```python
from build123d import *

# Parameters (mm, degrees)
SKETCH_1_R          = 1.75
EXTRUDE_1_DEPTH     = 5
CUT_EXTRUDE_1_REACH = 7
SKETCH_2_W          = 35
SKETCH_2_H          = 3
SKETCH_3_W          = 8
SKETCH_3_H          = 8
CUT_EXTRUDE_3_DEPTH = 6


with BuildPart() as part:
    # 草圖1 → 填料-伸長1 (new body)
    with BuildSketch(Plane.XY):
        Polygon((-30, 16.5), (-30, 8.5), (-22, 8.5), (-22, -8.5), (-30, -8.5), (-30, -16.5), (30, -16.5), (30, -8.5), (22, -8.5), (22, 8.5), (30, 8.5), (30, 16.5), align=None)
        with Locations((-26, 12.5)):
            Circle(SKETCH_1_R, mode=Mode.SUBTRACT)
        with Locations((26, 12.5)):
            Circle(SKETCH_1_R, mode=Mode.SUBTRACT)
        with Locations((-26, -12.5)):
            Circle(SKETCH_1_R, mode=Mode.SUBTRACT)
        with Locations((26, -12.5)):
            Circle(SKETCH_1_R, mode=Mode.SUBTRACT)
    extrude(amount=EXTRUDE_1_DEPTH)

    # 草圖2 → 除料-伸長1 (cut, up to next)
    with BuildSketch(Plane.XY.offset(5), mode=Mode.PRIVATE) as cut_extrude_1_sk1:
        with Locations((0, -7)):
            Rectangle(SKETCH_2_W, SKETCH_2_H)
    cut_extrude_1_tool1 = extrude(cut_extrude_1_sk1.sketch, amount=-CUT_EXTRUDE_1_REACH, mode=Mode.PRIVATE) & part.part
    add(cut_extrude_1_tool1.solids().sort_by_distance((0, -7, 5))[0], mode=Mode.SUBTRACT)

    # 草圖3 → 除料-伸長3 (cut, through all)
    with BuildSketch(Plane.XY):
        with Locations((26, -12.5)):
            Rectangle(SKETCH_3_W, SKETCH_3_H)
    extrude(amount=CUT_EXTRUDE_3_DEPTH, mode=Mode.SUBTRACT)


solid = part.part
```
Design review of the part built by this model. Coordinates are the model's own, in mm. A direction names the side the tool comes from. Give positions to 0.01 mm unless a question says otherwise; leave off trailing zeros. Write each loop counter-clockwise with the first axis right and the second up, starting at its lowest first coordinate (ties: lowest second). Pieces come first, ordered by that corner, then holes.
(1) Add section D-D (x = 11). Give the boundary of the cut face in (y, z), and give its area (3 significant figures).
Checked values:
outline: (-16.5, 0) - (-8.5, 0) - (-8.5, 5) - (-16.5, 5) - close; (-5.5, 0) - (16.5, 0) - (16.5, 5) - (-5.5, 5) - close
area: 150 mm2
(2) Add section C-C (z = 0.55). Give the boundary of the cut face in (x, y).
Checked values:
outline: (-30, -16.5) - (22, -16.5) - (22, 8.5) - (30, 8.5) - (30, 16.5) - (-30, 16.5) - (-30, 8.5) - (-22, 8.5) - (-22, -8.5) - (-30, -8.5) - close; hole circle Ø3.5 at (-26, -12.5); hole circle Ø3.5 at (-26, 12.5); hole (-17.5, -8.5) - (17.5, -8.5) - (17.5, -5.5) - (-17.5, -5.5) - close; hole circle Ø3.5 at (26, 12.5)
(3) Add section B-B (x = -26). Give the boundary of the cut face in (y, z).
Checked values:
outline: (-16.5, 0) - (-14.25, 0) - (-14.25, 5) - (-16.5, 5) - close; (-10.75, 0) - (-8.5, 0) - (-8.5, 5) - (-10.75, 5) - close; (8.5, 0) - (10.75, 0) - (10.75, 5) - (8.5, 5) - close; (14.25, 0) - (16.5, 0) - (16.5, 5) - (14.25, 5) - close
(4) Tool access review of faces 5 (the face through (-30, 13, 2)), 6 (the face through (0, 0, 0)), 7 (the face through (-22, 0, 2)), 8 (the face through (-17.5, -7, 3)), 9 (the face through (22, -4, 2)): name each direction out of +Z, -Z, +X, -X, +Y, -Y from which nothing blocks a thin tool from reaching the whole face with its end or side.
Checked values:
face 5: +Z, -Z, -X, +Y, -Y
face 6: -Z, +X, -X, +Y, -Y
face 7: +Z, -Z, -X
face 8: +Z, -Z
face 9: +Z, -Z, +X, -Y
(5) Wall thickness on line 1 along Y through (x, z) = (-26, 1.7); line 2 along Y through (x, z) = (-23.5, 3.55); line 3 along Y through (x, z) = (2, 1.75): over which ranges is each line inside the solid? List them lowest first.
Checked values:
line 1: y = -16.5 to -14.25, -10.75 to -8.5, 8.5 to 10.75, 14.25 to 16.5
line 2: y = -16.5 to -8.5, 8.5 to 16.5
line 3: y = -16.5 to -8.5, -5.5 to 16.5
(6) Add section A-A (y = -12.5). Give the boundary of the cut face in (x, z), and give its area (4 significant figures).
Checked values:
outline: (-30, 0) - (-27.75, 0) - (-27.75, 5) - (-30, 5) - close; (-24.25, 0) - (22, 0) - (22, 5) - (-24.25, 5) - close
area: 242.5 mm2
(7) Mouldability with a two-part tool opening along Y and no side actions: class faces 1 (the face through (0, 16.5, 2)), 2 (the face through (0, 0, 5)), 3 (the face through (0, -5.5, 3)), 4 (the face through (-4, -16.5, 2)) as +Y half, -Y half, draft (parallel to the pull), parting line (faces both ways), or undercut.
Checked values:
face 1: +Y half
face 2: draft
face 3: undercut
face 4: -Y half
(8) Clearance check with flat-ended pins moving along their axes: pin 1 Ø1 at (y, z) = (5.5, 0.5) entering from -X; pin 2 Ø3 at (x, y) = (26, 12.5) entering from -Z; pin 3 Ø1.5 at (y, z) = (-7.5, 2) entering from +X. State where each tip first meets the part, or that it passes through.
Checked values:
pin 1: stops at x = -22
pin 2: passes through
pin 3: stops at x = 22
